from build123d import *

# Parameters (mm, degrees)
PAD_DEPTH = 140


with BuildPart() as part:
    # Sketch → Pad (new body)
    with BuildSketch(Plane.XY):
        with BuildLine():
            Line((16.176132, 3), (-16.176132, 3))
            ThreePointArc((-16.176132, 3), (-17.195642, 2.600273), (-17.671784, 1.614134))
            Line((-17.671784, 1.614134), (-20.876825, -40.385866))
            ThreePointArc((-20.876825, -40.385866), (-20.481446, -41.519509), (-19.381173, -42))
            Line((-19.381173, -42), (-18, -42))
            Line((-18, -42), (-15.5, -9.239107))
            ThreePointArc((-5.52899, 0), (-12.32572, -2.664847), (-15.5, -9.239107))
            Line((-5.52899, 0), (5.52899, 0))
            ThreePointArc((15.5, -9.239107), (12.32572, -2.664847), (5.52899, 0))
            Line((15.5, -9.239107), (18, -42))
            Line((18, -42), (19.381173, -42))
            ThreePointArc((19.381173, -42), (20.481446, -41.519509), (20.876825, -40.385866))
            Line((20.876825, -40.385866), (17.671784, 1.614134))
            ThreePointArc((17.671784, 1.614134), (17.195642, 2.600273), (16.176132, 3))
        make_face()
    extrude(amount=PAD_DEPTH)


solid = part.part
Could you check a few things on this model? Use its own coordinates, in mm. A direction names the side the tool comes from. Coordinates: 2 decimals unless noted, no trailing zeros. Order: outer loops, then holes, each group sorted by start corner. A loop starts at its lowest first (then second) coordinate and runs counter-clockwise, first axis right, second up. Notation, with made-up numbers: (23, -32.75) -> (57, -32.75) arc R29 cw to (57, -11.75) -> close; hole circle Ø11 at (-28.5, 63). An arc over 180 degrees is marked (long way). One line per item, written item: value. Start each with the question number.
1) Which directions (+Z, -Z, +X, -X, +Y, -Y) give clear straight access to the entire face, cutting with the end or side of a thin tool? Please do faces 4 (the cylindrical face through (-12.249, -2.594, 69.02)), 5 (the flat face through (0, 3, 69)).
2) Imagine slicing it at A-A on y = -5. List the corners of the cut face in (x, z) for me, plus the area to 3 significant figures.
3) I'm going to push flat-ended pins straight in: pin 1 (3 mm diameter, centred on y = -18, z = 25, fed in from +X); pin 2 (8 mm diameter, centred on y = -3.5, z = 17.5, fed in from +X); pin 3 (12 mm diameter, centred on x = 7, z = 37.5, fed in from -Y). Where does each tip first touch, or does it pass through?
4) If I drill on L1, parallel to X at y = -33, z = 11; L2, parallel to X at y = -28, z = 24; L3, parallel to Y at x = 3, z = 93.5, over which ranges is the centre line in solid material (lowest first)? Write a range as [from, to].
5) We'd pull the mould along Y, two halves only. Please class faces 1 (the flat face through (-19.25, -19.09, 69.02)), 2 (the flat face through (0, 1, 140)), 3 (the flat face through (16.732, -25.39, 69.02)): +Y half, -Y half, draft (parallel to the pull), parting line (faces both ways), or undercut.
6) Imagine slicing it at D-D on y = -18. List the corners of the cut face in (x, z) for me.
7) Imagine slicing it at C-C on x = 0. List the corners of the cut face in (y, z) for me.
8) Imagine slicing it at B-B on z = 38.5. List the corners of the cut face in (x, y) for me.
Answer list:
1. face 4: +Z, -Z, -Y
1. face 5: +Z, -Z, +X, -X, +Y
2. outline: (-18.18, 0) -> (-14.19, 0) -> (-14.19, 140) -> (-18.18, 140) -> close; (14.19, 0) -> (18.18, 0) -> (18.18, 140) -> (14.19, 140) -> close
2. area: 1,120 mm2
3. pin 1: stops at x = 19.28
3. pin 2: stops at x = 18.37
3. pin 3: stops at y = -3.35
4. L1: x = [-20.31, -17.31], [17.31, 20.31]
4. L2: x = [-19.93, -16.93], [16.93, 19.93]
4. L3: y = [0, 3]
5. face 1: +Y half
5. face 2: draft
5. face 3: -Y half
6. outline: (-19.17, 0) -> (-16.17, 0) -> (-16.17, 140) -> (-19.17, 140) -> close; (16.17, 0) -> (19.17, 0) -> (19.17, 140) -> (16.17, 140) -> close
7. outline: (0, 0) -> (3, 0) -> (3, 140) -> (0, 140) -> close
8. outline: (-20.88, -40.39) arc R1.5 ccw to (-19.38, -42) -> (-18, -42) -> (-15.5, -9.24) arc R10 cw to (-5.53, 0) -> (5.53, 0) arc R10 cw to (15.5, -9.24) -> (18, -42) -> (19.38, -42) arc R1.5 ccw to (20.88, -40.39) -> (17.67, 1.61) arc R1.5 ccw to (16.18, 3) -> (-16.18, 3) arc R1.5 ccw to (-17.67, 1.61) -> close
